```python
from build123d import *

# Parameters (mm, degrees)
BOSS_EXTRUDE1_DEPTH = 18
SKETCH4_R           = 2.1
CUT_EXTRUDE3_DEPTH  = 10


with BuildPart() as part:
    # Sketch1 → Boss-Extrude1 (new body)
    with BuildSketch(Plane(origin=(0, 0, 0), x_dir=(1, 0, 0), z_dir=(0, 1, 0))):
        with BuildLine():
            Line((-10, 0), (0, 0))
            Line((0, 0), (0, 56.712101031))
            Line((0, 56.712101031), (-31.43, 56.712101031))
            Line((-31.43, 56.712101031), (-31.43, 96.46))
            Line((-31.43, 96.46), (-36, 96.46))
            Line((-36, 96.46), (-36, 26))
            ThreePointArc((-36, 26), (-17.615223689, 18.384776311), (-10, 0))
        make_face()
    extrude(amount=BOSS_EXTRUDE1_DEPTH)

    # Sketch4 → Cut-Extrude3 (cut)
    with BuildSketch(Plane(origin=(-31.43, 0, 0), x_dir=(0, 0, -1), z_dir=(1, 0, 0))):
        with Locations((81.26, 7.5)):
            Circle(SKETCH4_R)
        with Locations((93.96, 7.5)):
            Circle(SKETCH4_R)
        with Locations((68.56, 7.5)):
            Circle(SKETCH4_R)
    extrude(amount=-CUT_EXTRUDE3_DEPTH, mode=Mode.SUBTRACT)


solid = part.part
```
Verification items for the finished model (mm, model axes). A direction names the side the tool comes from. Give positions to 0.01 mm unless a question says otherwise; leave off trailing zeros. Order: outer loops, then holes, each group sorted by start corner. A loop starts at its lowest first (then second) coordinate and runs counter-clockwise, first axis right, second up. Notation, with made-up numbers: (9.5, -26) - (62.5, -26) arc R34 cw to (62.5, 9) - close; hole circle Ø3 at (30, 66). An arc over 180 degrees is marked (long way). Answer as CSV lines item,"result". Start each with the question number.
Item 1: Mould release check, pull along Y, two halves, no side actions. Record for faces 1 (the face through (-18, 0, -38)), 2 (the face through (-33.68, 7.59, -91.86)), 3 (the face through (-31.43, 9, -76)): released by +Y, released by -Y, zero draft, split by the parting line, or undercut.
Item 2: Access from +Z, -Z, +X, -X, +Y, -Y to the whole of each face (thin tool, end or side, straight path). Record for faces 4 (the face through (-15, 9, -56.712)), 5 (the face through (-34, 9, -96.46)).
Item 3: Gauge pin test, flat ends, axial feed: pin 1 (2 mm diameter, centred on x = -18.5, y = 4, fed in from +Z); pin 2 (4 mm diameter, centred on x = -20, y = 7.5, fed in from -Z); pin 3 (3 mm diameter, centred on x = -13.5, y = 11, fed in from +Z). Record the tip position at first contact, or that the pin passes through.
Item 4: Material ranges on L1, parallel to Y at x = -34.7, z = -81.26; L2, parallel to Z at x = -3.5, y = 4.25; L3, parallel to X at y = 3.75, z = -82, recorded low to high.
Item 5: Section check D-D, the plane x = -7. Record the boundary of the cut face in (y, z), plus the area to 3 significant figures.
Item 6: Section check B-B, the plane y = 7.5. Record the boundary of the cut face in (x, z).
Item 7: Section check C-C, the plane y = 16.5. Record the boundary of the cut face in (x, z), plus the area to 3 significant figures.
Item 8: Section check A-A, the plane z = -81.26. Record the boundary of the cut face in (x, y).
Filled in:
1,face 1,"released by -Y"
1,face 2,"undercut"
1,face 3,"zero draft"
2,face 4,"-Z, +X, +Y, -Y"
2,face 5,"-Z, +X, -X, +Y, -Y"
3,pin 1,"z = -18.27"
3,pin 2,"z = -56.71"
3,pin 3,"z = -10"
4,L1,"0 to 5.4, 9.6 to 18"
4,L2,"-56.71 to 0"
4,L3,"-36 to -31.43"
5,outline,"(0, -56.71) - (18, -56.71) - (18, 0) - (0, 0) - close"
5,area,"1,020 mm^2"
6,outline,"(-36, -96.46) - (-31.43, -96.46) - (-31.43, -96.06) - (-36, -96.06) - close; (-36, -91.86) - (-31.43, -91.86) - (-31.43, -83.36) - (-36, -83.36) - close; (-36, -79.16) - (-31.43, -79.16) - (-31.43, -70.66) - (-36, -70.66) - close; (-36, -66.46) - (-31.43, -66.46) - (-31.43, -56.71) - (0, -56.71) - (0, 0) - (-10, 0) arc R26 cw to (-36, -26) - close"
7,outline,"(-36, -96.46) - (-31.43, -96.46) - (-31.43, -56.71) - (0, -56.71) - (0, 0) - (-10, 0) arc R26 cw to (-36, -26) - close"
7,area,"1,690 mm^2"
8,outline,"(-36, 0) - (-31.43, 0) - (-31.43, 5.4) - (-36, 5.4) - close; (-36, 9.6) - (-31.43, 9.6) - (-31.43, 18) - (-36, 18) - close"
